Geometry: final body of the model. Coordinates: model frame, mm. A direction names the side the tool comes from. Give positions to 0.01 mm unless a question says otherwise; leave off trailing zeros. Order: outer loops, then holes, each group sorted by start corner. A loop starts at its lowest first (then second) coordinate and runs counter-clockwise, first axis right, second up. Notation, with made-up numbers: (-32.5, 84) -> (-2.5, 84) arc R31 ccw to (-2.5, 116) -> close; hole circle Ø6 at (-8, 62.5). An arc over 180 degrees is marked (long way). One line per question, with ' | ' between items.
from build123d import *

# Parameters (mm, degrees)
SKETCH1_W                                  = 63.5
SKETCH1_H                                  = 139.7
BOSS_EXTRUDE1_DEPTH                        = 6.35
SKETCH3_W                                  = 63.5
SKETCH3_H                                  = 6.35
BOSS_EXTRUDE2_DEPTH                        = 38.1
BOSS_EXTRUDE3_DEPTH                        = 6.35
SKETCH7_R                                  = 1.85
CUT_EXTRUDE1_DEPTH                         = 92.139645599
SKETCH8_W                                  = 6.35
SKETCH8_H                                  = 43.18
BOSS_EXTRUDE4_DEPTH                        = 38.1
SKETCH9_W                                  = 40.64
SKETCH9_H                                  = 12.7
BOSS_EXTRUDE5_DEPTH                        = 6.35
SKETCH10_R                                 = 1.65
CUT_EXTRUDE2_DEPTH                         = 12
MIRROR2_AT_THE_SECOND_PLANE_COPY_1_SKETC_R = 1.65
MIRROR2_AT_THE_SECOND_PLANE_COPY_1_DEPTH   = 12


with BuildPart() as part:
    # Sketch1 → Boss-Extrude1 (new body)
    with BuildSketch(Plane(origin=(0, 0, 0), x_dir=(1, 0, 0), z_dir=(0, 1, 0))):
        with Locations((-6.35, 0)):
            Rectangle(SKETCH1_W, SKETCH1_H)
    extrude(amount=BOSS_EXTRUDE1_DEPTH)

    # Sketch3 → Boss-Extrude2 (add)
    with BuildSketch(Plane(origin=(0, 6.35, 0), x_dir=(1, 0, 0), z_dir=(0, 1, 0))):
        with Locations((-6.35, 66.675)):
            Rectangle(SKETCH3_W, SKETCH3_H)
        with Locations((-6.35, -66.675)):
            Rectangle(SKETCH3_W, SKETCH3_H)
    extrude(amount=BOSS_EXTRUDE2_DEPTH)

    # Sketch6 → Boss-Extrude3 (add)
    with BuildSketch(Plane(origin=(0, 6.35, 0), x_dir=(1, 0, 0), z_dir=(0, 1, 0))):
        Polygon((25.4, 50.8), (31.75, 50.8), (31.75, 57.15), (38.1, 57.15), (38.1, 31.75), (31.75, 31.75), (31.75, 38.1), (25.4, 38.1), align=None)
    boss_extrude3 = extrude(amount=-BOSS_EXTRUDE3_DEPTH)

    # Mirror1: Boss-Extrude3 across plane
    add(boss_extrude3.mirror(Plane.XY))

    # Sketch7 → Cut-Extrude1 (cut, through all)
    with BuildSketch(Plane.XZ):
        with Locations(Location((-10.5, 0, 0), (0, 0, 270))):
            Circle(SKETCH7_R)
        with Locations(Location((-29.6, 0, 0), (0, 0, 270))):
            Circle(SKETCH7_R)
    extrude(amount=-CUT_EXTRUDE1_DEPTH, mode=Mode.SUBTRACT)

    # Sketch8 → Boss-Extrude4 (add)
    with BuildSketch(Plane(origin=(0, 6.35, 0), x_dir=(1, 0, 0), z_dir=(0, 1, 0))):
        with Locations((-34.925, 41.91)):
            Rectangle(SKETCH8_W, SKETCH8_H)
        with Locations((-34.925, -41.91)):
            Rectangle(SKETCH8_W, SKETCH8_H)
    extrude(amount=BOSS_EXTRUDE4_DEPTH)

    # Sketch9 → Boss-Extrude5 (add)
    with BuildSketch(Plane.ZY.offset(38.1)):
        with Locations((0, 38.1)):
            Rectangle(SKETCH9_W, SKETCH9_H)
    extrude(amount=-BOSS_EXTRUDE5_DEPTH)

    # Sketch10 → Cut-Extrude2 (cut)
    with BuildSketch(Plane(origin=(0, 44.45, 0), x_dir=(1, 0, 0), z_dir=(0, 1, 0))):
        with Locations(Location((-34.925, 66.675, 0), (0, 0, 270))):
            Circle(SKETCH10_R)
    cut_extrude2 = extrude(amount=-CUT_EXTRUDE2_DEPTH, mode=Mode.SUBTRACT)

    # Mirror2: Cut-Extrude2 across plane
    add(cut_extrude2.mirror(Plane.ZY.offset(6.35)), mode=Mode.SUBTRACT)

    # Mirror2 at the second plane: Cut-Extrude2 across plane
    add(cut_extrude2.mirror(Plane.XY), mode=Mode.SUBTRACT)

    # Mirror2 at the second plane copy 1 sketc → Mirror2 at the second plane copy 1 (cut)
    with BuildSketch(Plane(origin=(-12.7, 44.45, 0), x_dir=(-1, 0, 0), z_dir=(0, 1, 0))):
        with Locations(Location((-34.925, 66.675, 0), (0, 0, 270))):
            Circle(MIRROR2_AT_THE_SECOND_PLANE_COPY_1_SKETC_R)
    extrude(amount=-MIRROR2_AT_THE_SECOND_PLANE_COPY_1_DEPTH, mode=Mode.SUBTRACT)


solid = part.part
1) Section B-B on x = -10.5. Return loops of the section in (y, z), plus the area to 3 significant figures.
Check result:
outline: (0, -69.85) -> (44.45, -69.85) -> (44.45, -63.5) -> (6.35, -63.5) -> (6.35, -1.85) -> (0, -1.85) -> close; (0, 1.85) -> (6.35, 1.85) -> (6.35, 63.5) -> (44.45, 63.5) -> (44.45, 69.85) -> (0, 69.85) -> close | area: 1,350 mm^2
2) Section D-D on z = 24.5. Return loops of the section in (x, y), plus the area to 3 significant figures.
Check result:
outline: (-38.1, 0) -> (25.4, 0) -> (25.4, 6.35) -> (-31.75, 6.35) -> (-31.75, 44.45) -> (-38.1, 44.45) -> close | area: 645 mm^2
3) Set-up query: faces 4 (the flat face through (-35, 19, -20.32)), 5 (the flat face through (22, 32.45, 67)), 6 (the flat face through (-4, 25, 63.5)), 7 (the flat face through (35, 3, -31.75)), 8 (the flat face through (29, 3, 38.1)). Return all of +Z, -Z, +X, -X, +Y, -Y with unobstructed straight access to the full face (end or side cutting, diameter ignored); none if empty.
Check result:
face 4: +X, -X | face 5: +Y | face 6: +X, +Y | face 7: +X, +Y, -Y | face 8: +Y, -Y
4) Section A-A on z = 0. Return loops of the section in (x, y), plus the area to 3 significant figures.
Check result:
outline: (-38.1, 0) -> (-31.45, 0) -> (-31.45, 6.35) -> (-38.1, 6.35) -> close; (-38.1, 31.75) -> (-31.75, 31.75) -> (-31.75, 44.45) -> (-38.1, 44.45) -> close; (-27.75, 0) -> (-12.35, 0) -> (-12.35, 6.35) -> (-27.75, 6.35) -> close; (-8.65, 0) -> (25.4, 0) -> (25.4, 6.35) -> (-8.65, 6.35) -> close | area: 437 mm^2
5) Material intervals for probe 1 along Z at (x, y) = (-4.5, 14); probe 2 along X at (y, z) = (40, 59), sorted ascending. Write a range as from..to.
Check result:
probe 1: z = -69.85..-63.5, 63.5..69.85 | probe 2: x = -38.1..-31.75
6) Pull-direction query (X, two-part tool) for faces 1 (the flat face through (-31.75, 34, -1)), 2 (the flat face through (35, 3, 57.15)), 3 (the flat face through (-35, 32.45, -67)); classes: +X half, -X half, draft (parallel to the pull), parting line (faces both ways), or undercut.
Check result:
face 1: +X half | face 2: draft | face 3: undercut
7) Section C-C on y = 28. Return loops of the section in (x, z).
Check result:
outline: (-38.1, -69.85) -> (25.4, -69.85) -> (25.4, -63.5) -> (-31.75, -63.5) -> (-31.75, -20.32) -> (-38.1, -20.32) -> close; (-38.1, 20.32) -> (-31.75, 20.32) -> (-31.75, 63.5) -> (25.4, 63.5) -> (25.4, 69.85) -> (-38.1, 69.85) -> close
8) Contact query for flat-ended pins moving along their axis: pin 1 Ø7 at (x, y) = (29, 2) entering from +Z; pin 2 Ø1.6 at (x, z) = (21.5, 67) entering from +Y; pin 3 Ø6 at (x, z) = (-10.5, 0) entering from +Y. Output: stop coordinate, or through.
Check result:
pin 1: stops at z = 57.15 | pin 2: stops at y = 32.45 | pin 3: stops at y = 6.35
